```python
from build123d import *

# Parameters (mm, degrees)
ESBO_O1_W                = 143.01
ESBO_O1_H                = 54
RESSALTO_EXTRUS_O1_DEPTH = 10
ESBO_O14_W               = 2.7
ESBO_O14_H               = 57.87
RESSALTO_EXTRUS_O3_DEPTH = 143.01
ESBO_O2_R                = 16
CIRCULO_ROLAMENTO_DEPTH  = 19
ESBO_O7_R                = 10
CORTE_EXTRUS_O3_DEPTH    = 19
ESBO_O8_W                = 143.01
ESBO_O8_H                = 3.87
RESSALTO_EXTRUS_O2_DEPTH = 10
ESBO_O12_R               = 2.5
CORTE_EXTRUS_O6_DEPTH    = 17
CORTE_EXTRUS_O7_REACH    = 94.531
ESBO_O15_R               = 2.5


with BuildPart() as part:
    # Esboço1 → Ressalto-extrusão1 (new body)
    with BuildSketch(Plane.XY):
        Rectangle(ESBO_O1_W, ESBO_O1_H)
    extrude(amount=RESSALTO_EXTRUS_O1_DEPTH)

    # Esboço14 → Ressalto-extrusão3 (add)
    with BuildSketch(Plane.ZY.offset(71.505)):
        with Locations((-1.35, -1.935)):
            Rectangle(ESBO_O14_W, ESBO_O14_H)
    extrude(amount=-RESSALTO_EXTRUS_O3_DEPTH)

    # Esboço2 → Circulo rolamento (cut)
    with BuildSketch(Plane.XY.offset(10)):
        Circle(ESBO_O2_R)
    extrude(amount=-CIRCULO_ROLAMENTO_DEPTH, mode=Mode.SUBTRACT)

    # Esboço7 → Corte-extrusão3 (cut)
    with BuildSketch(Plane.XY.offset(10)):
        with Locations((-44.465, 0)):
            Circle(ESBO_O7_R)
        with Locations(Location((44.465, 0, 0), (0, 0, 90))):
            Circle(ESBO_O7_R)
    extrude(amount=-CORTE_EXTRUS_O3_DEPTH, mode=Mode.SUBTRACT)

    # Esboço8 → Ressalto-extrusão2 (add)
    with BuildSketch(Plane.XY.offset(10)):
        with Locations((0, -28.935)):
            Rectangle(ESBO_O8_W, ESBO_O8_H)
    extrude(amount=-RESSALTO_EXTRUS_O2_DEPTH)

    # Esboço12 → Corte-extrusão6 (cut)
    with BuildSketch(Plane.XZ.offset(30.87)):
        with Locations(Location((-61.505, 3.65, 0), (0, 0, 270))):
            Circle(ESBO_O12_R)
        with Locations(Location((61.505, 3.65, 0), (0, 0, 90))):
            Circle(ESBO_O12_R)
        with Locations(Location((0, 3.65, 0), (0, 0, 270))):
            Circle(ESBO_O12_R)
        with Locations(Location((-33.505, 3.65, 0), (0, 0, 270))):
            Circle(ESBO_O12_R)
        with Locations(Location((33.505, 3.65, 0), (0, 0, 90))):
            Circle(ESBO_O12_R)
    extrude(amount=-CORTE_EXTRUS_O6_DEPTH, mode=Mode.SUBTRACT)

    # Esboço15 → Corte-extrusão7 (cut, up to next)
    with BuildSketch(Plane(origin=(0, 27, 0), x_dir=(1, 0, 0), z_dir=(0, 1, 0)), mode=Mode.PRIVATE) as corte_extrus_o7_sk1:
        with Locations(Location((-44.505, -3.65, 0), (0, 0, 270))):
            Circle(ESBO_O15_R)
    corte_extrus_o7_tool1 = extrude(corte_extrus_o7_sk1.sketch, amount=-CORTE_EXTRUS_O7_REACH, mode=Mode.PRIVATE) & part.part
    # Esboço15 → Corte-extrusão7 (cut, up to next)
    with BuildSketch(Plane(origin=(0, 27, 0), x_dir=(1, 0, 0), z_dir=(0, 1, 0)), mode=Mode.PRIVATE) as corte_extrus_o7_sk2:
        with Locations(Location((44.505, -3.65, 0), (0, 0, 270))):
            Circle(ESBO_O15_R)
    corte_extrus_o7_tool2 = extrude(corte_extrus_o7_sk2.sketch, amount=-CORTE_EXTRUS_O7_REACH, mode=Mode.PRIVATE) & part.part
    add(corte_extrus_o7_tool1.solids().sort_by_distance((-44.505, 27, 3.65))[0], mode=Mode.SUBTRACT)
    add(corte_extrus_o7_tool2.solids().sort_by_distance((44.505, 27, 3.65))[0], mode=Mode.SUBTRACT)


solid = part.part
```
The listing builds one solid part. Answer for the finished solid, in the listing's coordinates (mm). A direction names the side the tool comes from. Round coordinates to 2 decimals unless told otherwise and drop trailing zeros. Order: outer loops, then holes, each group sorted by start corner. A loop starts at its lowest first (then second) coordinate and runs counter-clockwise, first axis right, second up. Notation, with made-up numbers: (33, 13) -> (67, 13) arc R16 cw to (67, 43) -> close; hole circle Ø7 at (60, -19.5). An arc over 180 degrees is marked (long way). Answer as CSV lines item,"result".
Q1. For a pull along Z with two mould halves and no side action, classify faces 4 (the flat face through (-17, -2, -2.7)), 5 (the flat face through (-17, -2, 10)), 6 (the flat face through (-1, 27, 4)), 7 (the flat face through (61, -13.87, 4)) as +Z half, -Z half, draft (parallel to the pull), parting line (faces both ways), or undercut.
Computed values:
face 4,"-Z half"
face 5,"+Z half"
face 6,"draft"
face 7,"undercut"
Q2. A cutting plane is placed at A-A on y = 0. Determine the outline of the cut face in (x, z) (3 decimals), plus the area to 3 significant figures.
Computed values:
outline,"(-71.505, -2.7) -> (-54.465, -2.7) -> (-54.465, 10) -> (-71.505, 10) -> close; (-34.465, -2.7) -> (-16, -2.7) -> (-16, 10) -> (-34.465, 10) -> close; (16, -2.7) -> (34.465, -2.7) -> (34.465, 10) -> (16, 10) -> close; (54.465, -2.7) -> (71.505, -2.7) -> (71.505, 10) -> (54.465, 10) -> close"
area,"902 mm^2"
Q3. Which of the six approach directions +Z, -Z, +X, -X, +Y, -Y give full straight-line access (tool end or side, diameter ignored) to faces 1 (the cylindrical face through (46.984, 18.457, 3.325)), 2 (the cylindrical face through (35.946, -22.489, 3.108)), 3 (the flat face through (-71.505, -2, 4))?
Computed values:
face 1,"+Y"
face 2,"-Y"
face 3,"+Z, -Z, -X, +Y, -Y"
Q4. A cutting plane is placed at C-C on y = 13.5. Determine the outline of the cut face in (x, z) (3 decimals), plus the area to 3 significant figures.
Computed values:
outline,"(-71.505, -2.7) -> (-8.588, -2.7) -> (-8.588, 10) -> (-71.505, 10) -> close; (8.588, -2.7) -> (71.505, -2.7) -> (71.505, 10) -> (8.588, 10) -> close; hole circle Ø5 at (-44.505, 3.65); hole circle Ø5 at (44.505, 3.65)"
area,"1,560 mm^2"
Q5. Consider line 1 (X direction, y = -26, z = 3.65) (3 decimals); line 2 (X direction, y = -9, z = 6.5) (3 decimals); line 3 (Z direction, x = 0, y = -26). Determine where each line is inside the solid, lowest interval first. Write a range as from..to.
Computed values:
line 1,"x = -71.505..-64.005, -59.005..-36.005, -31.005..-2.5, 2.5..31.005, 36.005..59.005, 64.005..71.505"
line 2,"x = -71.505..-48.824, -40.106..-13.229, 13.229..40.106, 48.824..71.505"
line 3,"z = -2.7..1.15, 6.15..10"
Q6. A cutting plane is placed at D-D on z = 8.75. Determine the outline of the cut face in (x, y) (3 decimals), plus the area to 3 significant figures.
Computed values:
outline,"(-71.505, -30.87) -> (71.505, -30.87) -> (71.505, 27) -> (-71.505, 27) -> close; hole circle Ø20 at (-44.465, 0); hole circle Ø32 at (0, 0); hole circle Ø20 at (44.465, 0)"
area,"6,840 mm^2"
Q7. Given pin 1 (4.5 mm diameter, centred on x = 33.505, z = 3.65, fed in from -Y); pin 2 (18 mm diameter, centred on x = 44.465, y = 0, fed in from -Z), each flat-ended and moving along its own axis, determine where each tip first touches the part or whether it passes through.
Computed values:
pin 1,"stops at y = -13.87"
pin 2,"passes through"
Q8. A cutting plane is placed at B-B on x = 0. Determine the outline of the cut face in (y, z), plus the area to 3 significant figures.
Computed values:
outline,"(-30.87, -2.7) -> (-16, -2.7) -> (-16, 1.15) -> (-30.87, 1.15) -> close; (-30.87, 6.15) -> (-16, 6.15) -> (-16, 10) -> (-30.87, 10) -> close; (16, -2.7) -> (27, -2.7) -> (27, 10) -> (16, 10) -> close"
area,"254 mm^2"
